Can you work these out from the model? Positions are in its coordinate system, mm. Face numbers are marked on the shaded views. A direction names the side the tool comes from. Round coordinates to 2 decimals unless told otherwise and drop trailing zeros. Order: outer loops, then holes, each group sorted by start corner. A loop starts at its lowest first (then second) coordinate and runs counter-clockwise, first axis right, second up. Notation, with made-up numbers: (82.25, 41) -> (114.25, 41) arc R23 ccw to (114.25, 78) -> close; hole circle Ø5 at (-30.5, 80.5). An arc over 180 degrees is marked (long way). One line per item, written item: value.
Autodesk Inventor part; units mm, degrees
ref_plane "YZ Plane" through (0, 0, 0) normal (1, 0, 0) x (0, 1, 0)
ref_plane "XZ Plane" through (0, 0, 0) normal (0, 1, 0) x (-1, 0, 0)
ref_plane "XY Plane" through (0, 0, 0) normal (0, 0, 1) x (1, 0, 0)
sketch "Sketch1" plane through (0, 0, 0) normal (0, 0, 1) x (1, 0, 0)
  circle A0 centre (-126.3, 8.5) radius 0.95
  circle A1 centre (-126.3, -8.5) radius 0.95
  circle A2 centre (-15.7, -8.5) radius 0.95
  circle A3 centre (-15.7, 8.5) radius 0.95
  line L0 (-21, 18) -> (-21, -18)
  line L1 (-121, -18) -> (-121, 18)
  line L2 (-121, 0) -> (-21, 0)
  line L3 (-126, 5) -> (-126, -5)
  line L4 (-126, -5) -> (-16, -5)
  line L5 (-16, -5) -> (-16, 5)
  line L6 (-16, 5) -> (-126, 5)
  line L7 (-126, 5) -> (-16, -5) construction
  line L8 (-126, -5) -> (-16, 5) construction
  line L9 (-126.3, 8.5) -> (-126.3, -8.5) construction
  line L10 (-129.3, 8.5) -> (-129.3, -8.5)
  line L11 (-123.3, -8.5) -> (-123.3, 8.5)
  arc A4 (-123.3, 8.5) -> (-129.3, 8.5) centre (-126.3, 8.5) ccw
  arc A5 (-129.3, -8.5) -> (-123.3, -8.5) centre (-126.3, -8.5) ccw
  line L12 (-15.7, 8.5) -> (-15.7, -8.5) construction
  line L13 (-18.7, 8.5) -> (-18.7, -8.5)
  line L14 (-12.7, -8.5) -> (-12.7, 8.5)
  arc A6 (-12.7, 8.5) -> (-18.7, 8.5) centre (-15.7, 8.5) ccw
  arc A7 (-18.7, -8.5) -> (-12.7, -8.5) centre (-15.7, -8.5) ccw
  line L15 (-16, 5) -> (-12.7, 8.5)
  line L16 (-16, -5) -> (-12.7, -8.5)
  line L17 (-126, 5) -> (-129.3, 8.5)
  line L18 (-126, -5) -> (-129.3, -8.5)
  point P0 (0, 0)
  point P1 (-71, 0)
  point P2 (-126.3, 0)
  point P3 (-15.7, 0)
  point P4 (-123.3, 5)
  point P5 (-123.3, -5)
  point P6 (-18.7, -5)
  point P7 (-18.7, 5)
  dimension "d0" = 10
  dimension "d1" = 110
  dimension "d2" = 6
  dimension "d3" = 6
extrude "Extrusion1" add sketch "Sketch1" along normal blind 3 contours L6 L13 L4 L0 | L0 L2 L1 L6 | L0 L4 L1 L2 | L13 A6 L15 L6 | L6 L5 L4 L13 | L1 L4 L11 L6 | L4 L16 A7 L13 | L11 L4 L3 L6 | L6 L17 A4 L11 | L11 A5 L18 L4
fillet "Fillet1" radius 8 4 edges at (-123.3, 5, 1.5) (-123.3, -5, 1.5) (-18.7, -5, 1.5) (-18.7, 5, 1.5)
fillet "Fillet2" radius 3 4 edges at (-126, 5, 1.5) (-126, -5, 1.5) (-16, 5, 1.5) (-16, -5, 1.5)
sketch "Sketch2" plane through (0, 0, 3) normal (0, 0, 1) x (1, 0, 0)
  arc A0 (-18.4375, -9.7273) -> (-12.7, -8.5) centre (-15.7, -8.5) ccw
  line L0 (-12.7, -8.5) -> (-15.1828, -5.8668)
  arc A1 (-16, -3.8087) -> (-15.1828, -5.8668) centre (-13, -3.8087) ccw
  line L1 (-16, -3.8087) -> (-16, 3.8087)
  arc A2 (-15.1828, 5.8668) -> (-16, 3.8087) centre (-13, 3.8087) ccw
  line L2 (-15.1828, 5.8668) -> (-12.7, 8.5)
  arc A3 (-12.7, 8.5) -> (-18.4375, 9.7273) centre (-15.7, 8.5) ccw
  arc A4 (-25.7374, 5) -> (-18.4375, 9.7273) centre (-25.7374, 13) ccw
  line L3 (-25.7374, 5) -> (-116.2626, 5)
  arc A5 (-123.5625, 9.7273) -> (-116.2626, 5) centre (-116.2626, 13) ccw
  arc A6 (-123.5625, 9.7273) -> (-129.3, 8.5) centre (-126.3, 8.5) ccw
  line L4 (-129.3, 8.5) -> (-126.8172, 5.8668)
  arc A7 (-126, 3.8087) -> (-126.8172, 5.8668) centre (-129, 3.8087) ccw
  line L5 (-126, 3.8087) -> (-126, -3.8087)
  arc A8 (-126.8172, -5.8668) -> (-126, -3.8087) centre (-129, -3.8087) ccw
  line L6 (-126.8172, -5.8668) -> (-129.3, -8.5)
  arc A9 (-129.3, -8.5) -> (-123.5625, -9.7273) centre (-126.3, -8.5) ccw
  arc A10 (-116.2626, -5) -> (-123.5625, -9.7273) centre (-116.2626, -13) ccw
  line L7 (-116.2626, -5) -> (-25.7374, -5)
  arc A11 (-18.4375, -9.7273) -> (-25.7374, -5) centre (-25.7374, -13) ccw
  circle A12 centre (-15.7, 8.5) radius 0.95
  circle A13 centre (-15.7, -8.5) radius 0.95
  circle A14 centre (-126.3, -8.5) radius 0.95
  circle A15 centre (-126.3, 8.5) radius 0.95
  line L8 (-126, 3.8087) -> (-126, -3.8087)
  line L9 (-126, 0) -> (-16, 0)
  line L10 (-126, 1) -> (-126, -1)
  line L11 (-126, -1) -> (-16, -1)
  line L12 (-16, -1) -> (-16, 1)
  line L13 (-16, 1) -> (-126, 1)
  line L14 (-126, 1) -> (-16, -1) construction
  line L15 (-126, -1) -> (-16, 1) construction
  line L16 (-16, -3.8087) -> (-16, 3.8087)
  point P0 (0, 0)
  point P1 (-71, 0)
  dimension "d8" = 2
extrude "Extrusion2" add sketch "Sketch2" along normal blind 5 contours L11 L5 L9 L1 | L9 L5 L13 L1
fillet "Fillet3" radius 1 2 edges at (-71, -1, 3) (-71, 1, 3)
fillet "Fillet4" radius 2 2 edges at (-126, 0, 8) (-16, 0, 8)
properties part number "test_bridge_1"
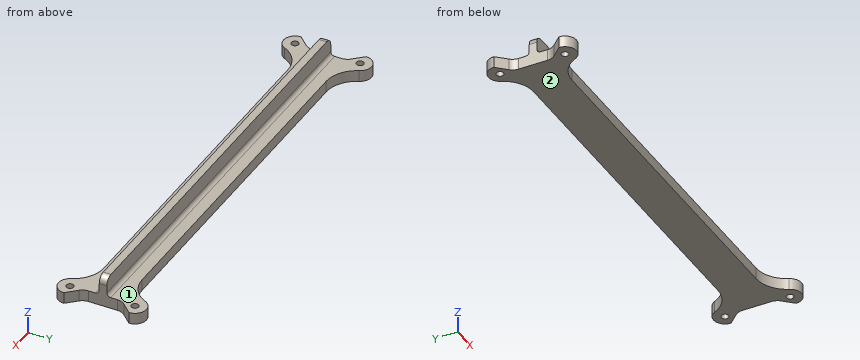
Q1. I want a section at C-C on y = 0. List the corners of the cut face in (x, z) for me.
Answers below:
outline: (-126, 0) -> (-16, 0) -> (-16, 6) arc R2 ccw to (-18, 8) -> (-124, 8) arc R2 ccw to (-126, 6) -> close
Q2. Will these pins go through, and if not, where does the flat tip stop? pin 1 Ø1.5 at (x, z) = (-81, 1.5) entering from -Y; pin 2 Ø2 at (y, z) = (-6, 1.5) entering from -X; pin 3 Ø1.5 at (y, z) = (3.5, 3) entering from -X; pin 4 Ø1.5 at (x, y) = (-66.5, 2) entering from -Z.
Answers below:
pin 1: y = -5
pin 2: x = -127.89
pin 3: x = -126.03
pin 4: z = 0
Q3. On a 3-axis mill with a long thin cutter (end or side, diameter ignored), from which of +Z, -Z, +X, -X, +Y, -Y can I reach the whole of each face in a straight line? I mean the marked faces 1 and 2. Say none if no direction works.
Answers below:
face 1: +Z, +X, -X, +Y
face 2: -Z, +X, -X, +Y, -Y
Q4. Please list where these lines run through material, in increasing order: line 1 along Y through (x, z) = (-126.3, 1.2); line 2 along Y through (x, z) = (-46.5, 6); line 3 along Y through (x, z) = (-37, 1.5).
Answers below:
line 1: -11.5 to -9.45, -7.55 to -5.12, 5.12 to 7.55, 9.45 to 11.5
line 2: -1 to 1
line 3: -5 to 5
Q5. I want a section at B-B on z = 1. Give the number of separate pieces and of enclosed holes in the cut face, plus the area to 3 significant figures.
Answers below:
separate pieces: 1
enclosed holes: 4
area: 1,240 mm^2
Q6. I want a section at A-A on x = -114. List the corners of the cut face in (y, z) for me.
Answers below:
outline: (-5, 0) -> (5, 0) -> (5, 3) -> (2, 3) arc R1 cw to (1, 4) -> (1, 8) -> (-1, 8) -> (-1, 4) arc R1 cw to (-2, 3) -> (-5, 3) -> close
